from build123d import *

# Parameters (mm, degrees)
F0_R     = 19.05
F1_DEPTH = 31.75
F3_DEPTH = 43.06758
F4_DEPTH = 25.4
F5_DEPTH = 4.7752
F6_DEPTH = 4.7752
F2_R     = 5.5626
F7_DEPTH = 61.9262
F8_DEPTH = 4.7625


with BuildPart() as f1:
    # F0 (on Right) → F1 (new body, symmetric)
    with BuildSketch(Plane.YZ):
        with BuildLine():
            Line((38.1, 28.575), (0, 28.575))
            ThreePointArc((0, 28.575), (-27.3235693319, -8.3638020041), (15.9950252975, -23.6788891364))
            ThreePointArc((15.9950252975, -23.6788891364), (25.7719232537, -12.3425522809), (28.4756083945, 2.38125))
            ThreePointArc((28.4756083945, 2.38125), (30.9572676717, 9.6234554837), (37.9674778593, 12.7))
            Line((37.9674778593, 12.7), (69.85, 12.7))
            Line((69.85, 12.7), (101.7325221407, 12.7))
            Line((101.7325221407, 12.7), (101.7325221407, 33.3502))
            Line((101.7325221407, 33.3502), (38.1, 33.3502))
            Line((38.1, 33.3502), (38.1, 28.575))
        make_face()
        Circle(F0_R, mode=Mode.SUBTRACT)
    extrude(amount=F1_DEPTH, both=True)

    # F2 (on face) → F3 (cut)
    with BuildSketch(Plane.XY.offset(33.3502)):
        with BuildLine():
            ThreePointArc((30.4170945511, 56.4638468789), (31.4122833813, 53.7092867856), (31.75, 50.8))
            Line((31.75, 50.8), (31.75, 101.7325221407))
            Line((31.75, 101.7325221407), (-1.274e-07, 101.7325221407))
            ThreePointArc((-1.274e-07, 101.7325221407), (6.6842779412, 99.8311529985), (11.3670945511, 94.6963690195))
            Line((11.3670945511, 94.6963690195), (30.4170945511, 56.4638468789))
        make_face()
    extrude(amount=-F3_DEPTH, mode=Mode.SUBTRACT)

    # F2 (on face) → F4 (cut)
    with BuildSketch(Plane.XY.offset(33.3502)):
        with BuildLine():
            Line((-31.75, 101.7325221407), (-31.75, 50.8))
            ThreePointArc((-31.75, 50.8), (-31.4122833813, 53.7092867856), (-30.4170945511, 56.4638468789))
            Line((-30.4170945511, 56.4638468789), (-11.3670945511, 94.6963690195))
            ThreePointArc((-11.3670945511, 94.6963690195), (-6.6842780495, 99.8311529315), (-1.274e-07, 101.7325221407))
            Line((-1.274e-07, 101.7325221407), (-31.75, 101.7325221407))
        make_face()
    extrude(amount=-F4_DEPTH, mode=Mode.SUBTRACT)

    # F2 (on face) → F5 (cut)
    with BuildSketch(Plane.XY.offset(33.3502)):
        with BuildLine():
            Line((-31.75, 38.1), (-19.05, 38.1))
            ThreePointArc((-19.05, 38.1), (-28.0302561211, 41.8197438789), (-31.75, 50.8))
            Line((-31.75, 50.8), (-31.75, 38.1))
        make_face()
    extrude(amount=-F5_DEPTH, mode=Mode.SUBTRACT)

    # F2 (on face) → F6 (cut)
    with BuildSketch(Plane.XY.offset(33.3502)):
        with BuildLine():
            ThreePointArc((31.75, 50.8), (28.0302561211, 41.8197438789), (19.05, 38.1))
            Line((19.05, 38.1), (31.75, 38.1))
            Line((31.75, 38.1), (31.75, 50.8))
        make_face()
    extrude(amount=-F6_DEPTH, mode=Mode.SUBTRACT)

    # F2 (on face) → F7 (cut, through all)
    with BuildSketch(Plane.XY.offset(33.3502)):
        with Locations((-19.05, 50.8)):
            Circle(F2_R)
        with Locations((0, 84.1502)):
            Circle(F2_R)
        with Locations((19.05, 50.8)):
            Circle(F2_R)
    extrude(amount=-F7_DEPTH, mode=Mode.SUBTRACT)

    # F0 (on Right) → F8 (join, symmetric)
    with BuildSketch(Plane.YZ):
        with BuildLine():
            ThreePointArc((28.4756083945, 2.38125), (25.7719232537, -12.3425522809), (15.9950252975, -23.6788891364))
            Line((15.9950252975, -23.6788891364), (69.85, 12.7))
            Line((69.85, 12.7), (37.9674778593, 12.7))
            ThreePointArc((37.9674778593, 12.7), (30.9572676717, 9.6234554837), (28.4756083945, 2.38125))
        make_face()
    extrude(amount=F8_DEPTH, both=True)


solid = f1.part
CAD build for the part. Positions are in the model's coordinates, mm. A direction names the side the tool comes from. Round coordinates to 2 decimals unless told otherwise and drop trailing zeros. Write each loop counter-clockwise with the first axis right and the second up, starting at its lowest first coordinate (ties: lowest second). Pieces come first, ordered by that corner, then holes. Notation, with made-up numbers: M 73,77.25 L 116,77.25 A17 ccw 116,83.25 Z; hole C -25,-34.5 d4. An arc over 180 degrees is marked long. Put each result on its own line as item: value. Start each with the question number.
1) Saw through at C-C, the plane y = -8.5. Write the cut outline in (x, z), and give its area (3 significant figures).
2) Pull direction X, two halves, no side cores. Call faces 3 (the flat face through (0, 38.1, 31)), 4 (the flat face through (-31.75, 19, 7)), 5 (the cylindrical face through (21.617, 45.865, 23.17)), 6 (the cylindrical face through (-16.483, 45.865, 23.17)): pulls with the +X half, pulls with the -X half, needs draft (parallel to the pull), parting line crosses it, or undercut.
3) Saw through at D-D, the plane x = 2. Write the cut outline in (y, z) (3 decimals), and give its area (3 significant figures).
4) Saw through at A-A, the plane x = -21. Write the cut outline in (y, z) (3 decimals), and give its area (3 significant figures).
5) Drill centre lines: probe 1 along Z at (x, y) = (17, 0) (3 decimals); probe 2 along Y at (x, z) = (15.5, 17.5); probe 3 along X at (y, z) = (50, 26). Where is each one in solid material? Low to high. Write a range as [from, to].
6) Pin check, flat tips, straight feed: pin 1 Ø3 at (y, z) = (57.5, 8.5) entering from -X; pin 2 Ø1.4 at (x, z) = (9.5, 31.5) entering from -Y; pin 3 Ø6.5 at (x, y) = (-19.05, 50.8) entering from -Z; pin 4 Ø4 at (x, z) = (-23.5, 22) entering from +Y. Stop position of each tip, or through.
7) Saw through at B-B, the plane z = 5.5. Write the cut outline in (x, y).
8) 3-axis set-ups, long thin cutter, end or side, ignore diameter. For faces 1 (the flat face through (-7, 62, 12.7)), 2 (the flat face through (0, 63, 33.35)): which of +Z, -Z, +X, -X, +Y, -Y reach the whole face in a straight line?
Resolved:
1. outline: M -31.75,-27.28 L 31.75,-27.28 L 31.75,-17.05 L -31.75,-17.05 Z; M -31.75,17.05 L 31.75,17.05 L 31.75,27.28 L -31.75,27.28 Z
1. area: 1,300 mm²
2. face 3: needs draft
2. face 4: pulls with the -X half
2. face 5: undercut
2. face 6: undercut
3. outline: M 0,28.575 A28.575 ccw long 15.995,-23.679 L 69.85,12.7 L 78.96,12.7 L 78.96,33.35 L 38.1,33.35 L 38.1,28.575 Z; M 89.341,12.7 L 101.574,12.7 L 101.574,33.35 L 89.341,33.35 Z; hole C 0,0 d38.1
3. area: 3,460 mm²
4. outline: M 0,28.575 A28.575 ccw long 28.476,2.381 A9.525 cw 37.967,12.7 L 45.59,12.7 L 45.59,33.35 L 38.251,33.35 L 38.251,28.575 Z; M 56.01,12.7 L 75.364,12.7 L 75.364,33.35 L 56.01,33.35 Z; hole C 0,0 d38.1
4. area: 2,320 mm²
5. probe 1: [-28.575, -19.05], [19.05, 28.575]
5. probe 2: [-22.59, -7.53], [7.53, 46.52], [55.08, 86.4]
5. probe 3: [-31.75, -24.55], [-13.55, 13.55], [24.55, 31.75]
6. pin 1: x = -4.76
6. pin 2: y = 38.1
6. pin 3: through
6. pin 4: y = 74.36
7. outline: M -31.75,-28.04 L 31.75,-28.04 L 31.75,-18.24 L -31.75,-18.24 Z; M -31.75,18.24 L 31.75,18.24 L 31.75,28.73 L 4.76,28.73 L 4.76,59.19 L -4.76,59.19 L -4.76,28.73 L -31.75,28.73 Z
8. face 1: -Z, +Y
8. face 2: +Z, +X, -X, +Y, -Y
